from build123d import *

# Parameters (mm, degrees)
SKETCH2_W           = 38
SKETCH2_H           = 38
BOSS_EXTRUDE1_DEPTH = 20
CUT_EXTRUDE1_DEPTH  = 20
SKETCH7_R           = 2.25
CUT_EXTRUDE2_DEPTH  = 5


with BuildPart() as part:
    # Sketch2 → Boss-Extrude1 (new body)
    with BuildSketch(Plane(origin=(0, 0, 0), x_dir=(1, 0, 0), z_dir=(0, 1, 0))):
        Rectangle(SKETCH2_W, SKETCH2_H)
    extrude(amount=BOSS_EXTRUDE1_DEPTH)

    # Sketch3 → Cut-Extrude1 (cut)
    with BuildSketch(Plane(origin=(0, 20, 0), x_dir=(1, 0, 0), z_dir=(0, 1, 0))):
        Polygon((-19, 19), (19, -19), (19, 19), align=None)
    extrude(amount=-CUT_EXTRUDE1_DEPTH, mode=Mode.SUBTRACT)

    # Sketch7 → Cut-Extrude2 (cut)
    with BuildSketch(Plane(origin=(0, 0, 0), x_dir=(-1, 0, 0), z_dir=(0, -1, 0))):
        with Locations(Location((12.5, 0, 0), (0, 0, 90))):
            Circle(SKETCH7_R)
        with Locations(Location((0, -12.5, 0), (0, 0, 90))):
            Circle(SKETCH7_R)
    extrude(amount=-CUT_EXTRUDE2_DEPTH, mode=Mode.SUBTRACT)


solid = part.part
Build history of the part. All positions in model axes, mm. A direction names the side the tool comes from. Give positions to 0.01 mm unless a question says otherwise; leave off trailing zeros. Write each loop counter-clockwise with the first axis right and the second up, starting at its lowest first coordinate (ties: lowest second). Pieces come first, ordered by that corner, then holes. Notation, with made-up numbers: (51.25, 13.5) - (95.25, 13.5) arc R29 ccw to (95.25, 33.5) - close; hole circle Ø4 at (10.5, -24.5). An arc over 180 degrees is marked (long way). Use one line per item in the form item = value. Start each with the question number.
1. Drop flat-ended pins along their axis: pin 1 Ø6 at (x, y) = (4, 7.5) entering from -Z; pin 2 Ø3 at (x, y) = (5, 8) entering from -Z; pin 3 Ø10 at (x, y) = (-2.5, 4) entering from -Z. Give the stop position or say it passes through.
2. Band-saw the part on B-B on z = 0. Write the cut outline in (x, y).
3. Band-saw the part on A-A on y = 1.5. Write the cut outline in (x, z), plus the area to 3 significant figures.
4. Band-saw the part on C-C on x = 0. Write the cut outline in (y, z).
5. Band-saw the part on D-D on y = 15.5. Write the cut outline in (x, z), plus the area to 3 significant figures.
6. 3-axis set-ups, long thin cutter, end or side, ignore diameter. For faces 1 (the face through (-12, 5, 0)), 2 (the face through (0, 10, 0)): which of +Z, -Z, +X, -X, +Y, -Y reach the whole face in a straight line?
7. Probe line 1 (X direction, y = 1.8, z = 0); line 2 (X direction, y = 3.8, z = 12.5); line 3 (Y direction, x = -2, z = 12). List the from-to ranges inside material, lowest first. Write a range as [from, to].
8. Two-plate mould, pull along X, no slides. Class faces 3 (the face through (-9, 0, 8)), 4 (the face through (0, 5, 13)), 5 (the face through (-19, 10, 0)), 6 (the face through (-10.27, 2.46, 0.29)): released by +X, released by -X, zero draft, split by the parting line, or undercut.
Conclusion:
q1.pin_1 = 1
q1.pin_2 = 3.5
q1.pin_3 = -7.5
q2.outline = (-19, 0) - (-14.75, 0) - (-14.75, 5) - (-10.25, 5) - (-10.25, 0) - (0, 0) - (0, 20) - (-19, 20) - close
q3.outline = (-19, -19) - (19, 19) - (-19, 19) - close; hole circle Ø4.5 at (-12.5, 0); hole circle Ø4.5 at (0, 12.5)
q3.area = 690 mm²
q4.outline = (0, 0) - (20, 0) - (20, 19) - (0, 19) - (0, 14.75) - (5, 14.75) - (5, 10.25) - (0, 10.25) - close
q5.outline = (-19, -19) - (19, 19) - (-19, 19) - close
q5.area = 722 mm²
q6.face_1 = -Y
q6.face_2 = -Z, +X, +Y, -Y
q7.line_1 = [-19, -14.75], [-10.25, 0]
q7.line_2 = [-19, -2.25], [2.25, 12.5]
q7.line_3 = [5, 20]
q8.face_3 = zero draft
q8.face_4 = undercut
q8.face_5 = released by -X
q8.face_6 = undercut
